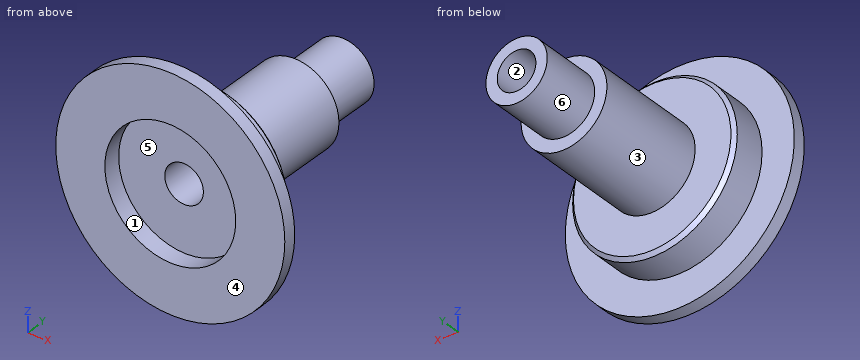
```python
from build123d import *

# Parameters (mm, degrees)
F0_R      = 60
F1_DEPTH  = 160
F2_R      = 115
F3_DEPTH  = 50
F4_R      = 160
F5_DEPTH  = 18
F6_SIZE   = 5
F7_R      = 42.875
F8_DEPTH  = 86
F9_R      = 27
F10_DEPTH = 430
F11_R     = 91.436725
F12_DEPTH = 25


with BuildPart() as f1:
    # F0 (on Front) → F1 (new body)
    with BuildSketch(Plane.XZ):
        Circle(F0_R)
    extrude(amount=F1_DEPTH)

    # F2 (on face) → F3 (join)
    with BuildSketch(Plane.XZ.offset(160)):
        Circle(F2_R)
    extrude(amount=F3_DEPTH)

    # F4 (on face) → F5 (join)
    with BuildSketch(Plane.XZ.offset(210)):
        Circle(F4_R)
    extrude(amount=F5_DEPTH)

    # F6
    f6_edges = [f1.edges().sort_by_distance(p)[0] for p in [
        (-115, -160, 0),
    ]]
    chamfer(f6_edges, length=F6_SIZE)

    # F7 (on face) → F8 (join)
    with BuildSketch(Plane(origin=(0, 0, 0), x_dir=(-1, 0, 0), z_dir=(0, 1, 0))):
        Circle(F7_R)
    extrude(amount=F8_DEPTH)

    # F9 (on face) → F10 (cut)
    with BuildSketch(Plane(origin=(0, 86, 0), x_dir=(-1, 0, 0), z_dir=(0, 1, 0))):
        Circle(F9_R)
    extrude(amount=-F10_DEPTH, mode=Mode.SUBTRACT)

    # F11 (on face) → F12 (cut)
    with BuildSketch(Plane.XZ.offset(228)):
        Circle(F11_R)
    extrude(amount=-F12_DEPTH, mode=Mode.SUBTRACT)


solid = f1.part
```
The model under review builds one solid part; all positions refer to its coordinate system, in mm. Face numbers are marked on the shaded views. A direction names the side the tool comes from. Round coordinates to 2 decimals unless told otherwise and drop trailing zeros. Write each loop counter-clockwise with the first axis right and the second up, starting at its lowest first coordinate (ties: lowest second). Pieces come first, ordered by that corner, then holes. Notation, with made-up numbers: (-13, 51.25) - (45, 51.25) arc R35 cw to (45, 83.25) - close; hole circle Ø4 at (13.5, 63). An arc over 180 degrees is marked (long way). Use one line per item in the form item = value.
Q1. Tool access review of the marked faces 1, 2 and 3: name each direction out of +Z, -Z, +X, -X, +Y, -Y from which nothing blocks a thin tool from reaching the whole face with its end or side.
Answer key:
face_1 = -Y
face_2 = +Y, -Y
face_3 = +Y
Q2. Consider section D-D (y = 47). State the section outline as (x, z) points (3 decimals), and give its area (3 significant figures).
Answer key:
outline = circle Ø85.75 at (0, 0); hole circle Ø54 at (0, 0)
area = 3,480 mm2
Q3. Consider section A-A (x = 0). State the section outline as (y, z) points (3 decimals), and give its area (3 significant figures).
Answer key:
outline = (-228, -160) - (-210, -160) - (-210, -115) - (-165, -115) - (-160, -110) - (-160, -60) - (0, -60) - (0, -42.875) - (86, -42.875) - (86, -27) - (-203, -27) - (-203, -91.437) - (-228, -91.437) - close; (-228, 91.437) - (-203, 91.437) - (-203, 27) - (86, 27) - (86, 42.875) - (0, 42.875) - (0, 60) - (-160, 60) - (-160, 110) - (-165, 115) - (-210, 115) - (-210, 160) - (-228, 160) - close
area = 23,600 mm2
Q4. Consider section B-B (z = 0). State the section outline as (x, y) points (3 decimals).
Answer key:
outline = (-160, -228) - (-91.437, -228) - (-91.437, -203) - (-27, -203) - (-27, 86) - (-42.875, 86) - (-42.875, 0) - (-60, 0) - (-60, -160) - (-110, -160) - (-115, -165) - (-115, -210) - (-160, -210) - close; (27, -203) - (91.437, -203) - (91.437, -228) - (160, -228) - (160, -210) - (115, -210) - (115, -165) - (110, -160) - (60, -160) - (60, 0) - (42.875, 0) - (42.875, 86) - (27, 86) - close
Q5. Consider section C-C (y = -28.5). State the section outline as (x, z) points.
Answer key:
outline = circle Ø120 at (0, 0); hole circle Ø54 at (0, 0)
Q6. Draft analysis for pull direction Z (two halves, no side actions). For the marked faces 4, 5 and 6, state which applies: +Z half, -Z half, draft (parallel to the pull), parting line (faces both ways), or undercut.
Answer key:
face_4 = draft
face_5 = undercut
face_6 = parting line
Q7. Insertion check: pin 1 Ø6 at (y, z) = (38, -26.5) entering from -X. The pin has a flat end and moves straight along its axis. Give the tip position at first contact, or say it passes through.
Answer key:
pin_1 = -35.86
Q8. For line 1 (Z direction, x = 0, y = -216.25); line 2 (Z direction, x = 0, y = -54.5); line 3 (Y direction, x = 6.5, z = -67.5), list the stretches that pass through material, from the lowest coordinate up. Write a range as [from, to].
Answer key:
line_1 = [-160, -91.44], [91.44, 160]
line_2 = [-60, -27], [27, 60]
line_3 = [-203, -160]
